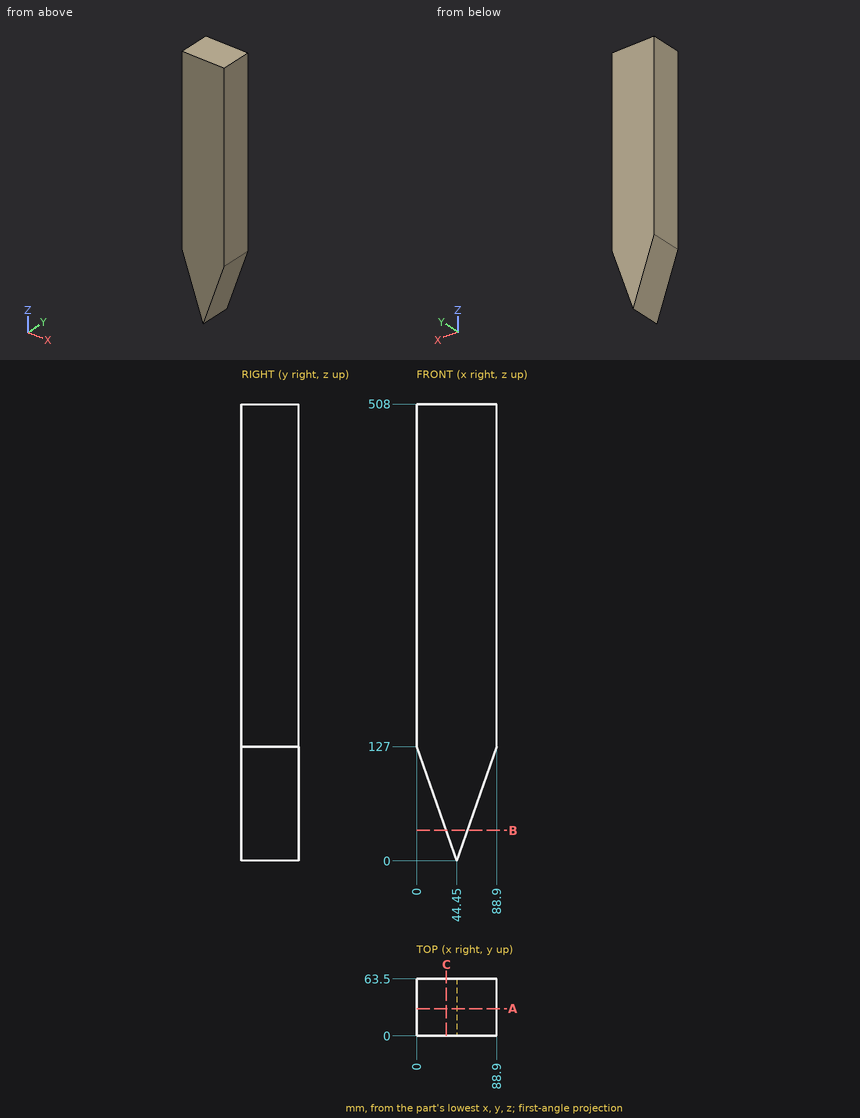
Geometry: see drawing. Coordinates: mm, zero at the bounding-box minimum. Give positions to 0.01 mm unless a question says otherwise; leave off trailing zeros. Write each loop counter-clockwise with the first axis right and the second up, starting at its lowest first coordinate (ties: lowest second). Pieces come first, ordered by that corner, then holes. Notation, with made-up numbers: M -7.75,-12 L 42.25,-12 A24 ccw 42.25,15 Z; hole C 24.5,-22 d7. An arc over 180 degrees is marked long. Answer as a JSON object with one key per item and string values.
Q1. Ray query, line 1 along X through (y, z) = (6, 81.5) (3 decimals). Return the intervals inside material, ascending.
Geometry check:
{"line 1": "x = 15.925 to 72.975"}
Q2. Cut plane B-B, the plane z = 34. Return the cut outline in (x, y), then the cut area to 3 significant figures.
Geometry check:
{"outline": "M 32.55,0 L 56.35,0 L 56.35,63.5 L 32.55,63.5 Z", "area": "1,510 mm^2"}
Q3. Cut plane A-A, the plane y = 30.5. Return the cut outline in (x, z), then the cut area to 3 significant figures.
Geometry check:
{"outline": "M 0,127 L 44.45,0 L 88.9,127 L 88.9,508 L 0,508 Z", "area": "39,500 mm^2"}
Q4. Cut plane C-C, the plane x = 33. Return the cut outline in (y, z), then the cut area to 3 significant figures.
Geometry check:
{"outline": "M 0,32.71 L 63.5,32.71 L 63.5,508 L 0,508 Z", "area": "30,200 mm^2"}
